Model file for the job. Use its own axes, mm. Give positions to 0.01 mm unless a question says otherwise; leave off trailing zeros. Write each loop counter-clockwise with the first axis right and the second up, starting at its lowest first coordinate (ties: lowest second). Pieces come first, ordered by that corner, then holes. Notation, with made-up numbers: (54.25, 40.5) - (92.25, 40.5) arc R32 ccw to (92.25, 74.5) - close; hole circle Ø10 at (12, 75.25). An arc over 180 degrees is marked (long way). Use CSV: the item, a comma, the result in double quotes.
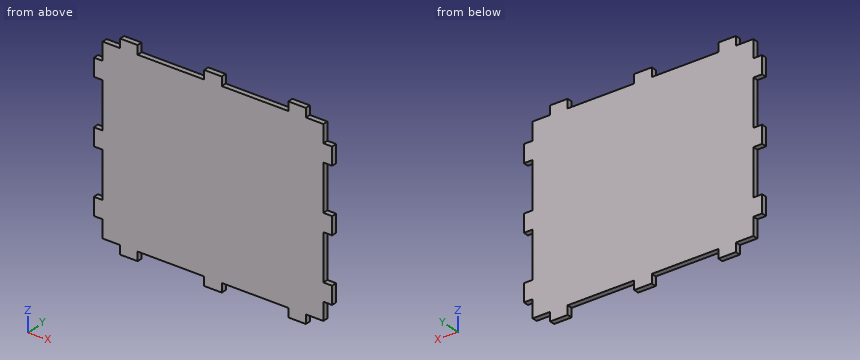
from build123d import *

# Parameters (mm, degrees)
F0_W     = 6.35
F0_H     = 12.7
F0_W_2   = 12.7
F0_H_2   = 6.35
F1_DEPTH = 3.81


# Not quite as in the source:
# - a feature names something its author has since deleted; it is built from what else it names


with BuildPart() as f1:
    # F0 (on Front) → F1 (new body)
    with BuildSketch(Plane.XZ):
        with Locations((-354.6769669852, 49.3793434303)):
            Rectangle(F0_W, F0_H)
        with Locations((-361.0269669852, 49.3793434303)):
            Rectangle(F0_W, F0_H)
        Polygon((-332.4519669852, -61.5706565697), (-284.2019669852, -61.5706565697), (-284.2019669852, -55.2206565697), (-277.8519669852, -55.2206565697), (-277.8519669852, 62.0793434303), (-284.2019669852, 62.0793434303), (-284.2019669852, 68.4293434303), (-332.4519669852, 68.4293434303), (-332.4519669852, 62.0793434303), (-345.1519669852, 62.0793434303), (-345.1519669852, 68.4293434303), (-357.8519669852, 68.4293434303), (-357.8519669852, 55.7293434303), (-351.5019669852, 55.7293434303), (-351.5019669852, 43.0293434303), (-357.8519669852, 43.0293434303), (-357.8519669852, 9.7793434303), (-351.5019669852, 9.7793434303), (-351.5019669852, -2.9206565697), (-357.8519669852, -2.9206565697), (-357.8519669852, -36.1706565697), (-351.5019669852, -36.1706565697), (-351.5019669852, -48.8706565697), (-357.8519669852, -48.8706565697), (-357.8519669852, -61.5706565697), (-345.1519669852, -61.5706565697), (-345.1519669852, -55.2206565697), (-332.4519669852, -55.2206565697), align=None)
        with Locations((-338.8019669852, 65.2543434303)):
            Rectangle(F0_W_2, F0_H_2)
        with Locations((-338.8019669852, 71.6043434303)):
            Rectangle(F0_W_2, F0_H_2)
        Polygon((-210.5519669852, -61.5706565697), (-197.8519669852, -61.5706565697), (-197.8519669852, -48.8706565697), (-204.2019669852, -48.8706565697), (-204.2019669852, -36.1706565697), (-197.8519669852, -36.1706565697), (-197.8519669852, -2.9206565697), (-204.2019669852, -2.9206565697), (-204.2019669852, 9.7793434303), (-197.8519669852, 9.7793434303), (-197.8519669852, 43.0293434303), (-204.2019669852, 43.0293434303), (-204.2019669852, 55.7293434303), (-197.8519669852, 55.7293434303), (-197.8519669852, 68.4293434303), (-210.5519669852, 68.4293434303), (-210.5519669852, 62.0793434303), (-223.2519669852, 62.0793434303), (-223.2519669852, 68.4293434303), (-271.5019669852, 68.4293434303), (-271.5019669852, 62.0793434303), (-277.8519669852, 62.0793434303), (-277.8519669852, -55.2206565697), (-271.5019669852, -55.2206565697), (-271.5019669852, -61.5706565697), (-223.2519669852, -61.5706565697), (-223.2519669852, -55.2206565697), (-210.5519669852, -55.2206565697), align=None)
        Polygon((-284.2019669852, 68.4293434303), (-277.8519669852, 68.4293434303), (-271.5019669852, 68.4293434303), (-271.5019669852, 74.7793434303), (-284.2019669852, 74.7793434303), align=None)
        with Locations((-274.6769669852, 65.2543434303)):
            Rectangle(F0_W, F0_H_2)
        with Locations((-281.0269669852, 65.2543434303)):
            Rectangle(F0_W, F0_H_2)
        with Locations((-216.9019669852, 71.6043434303)):
            Rectangle(F0_W_2, F0_H_2)
        with Locations((-216.9019669852, 65.2543434303)):
            Rectangle(F0_W_2, F0_H_2)
        with Locations((-354.6769669852, 3.4293434303)):
            Rectangle(F0_W, F0_H)
        with Locations((-361.0269669852, 3.4293434303)):
            Rectangle(F0_W, F0_H)
        with Locations((-361.0269669852, -42.5206565697)):
            Rectangle(F0_W, F0_H)
        with Locations((-338.8019669852, -64.7456565697)):
            Rectangle(F0_W_2, F0_H_2)
        with Locations((-354.6769669852, -42.5206565697)):
            Rectangle(F0_W, F0_H)
        with Locations((-338.8019669852, -58.3956565697)):
            Rectangle(F0_W_2, F0_H_2)
        with Locations((-281.0269669852, -58.3956565697)):
            Rectangle(F0_W, F0_H_2)
        with Locations((-274.6769669852, -58.3956565697)):
            Rectangle(F0_W, F0_H_2)
        Polygon((-271.5019669852, -67.9206565697), (-271.5019669852, -61.5706565697), (-277.8519669852, -61.5706565697), (-284.2019669852, -61.5706565697), (-284.2019669852, -67.9206565697), align=None)
        with Locations((-216.9019669852, -64.7456565697)):
            Rectangle(F0_W_2, F0_H_2)
        with Locations((-216.9019669852, -58.3956565697)):
            Rectangle(F0_W_2, F0_H_2)
        with Locations((-201.0269669852, -42.5206565697)):
            Rectangle(F0_W, F0_H)
        with Locations((-194.6769669852, -42.5206565697)):
            Rectangle(F0_W, F0_H)
        with Locations((-201.0269669852, 3.4293434303)):
            Rectangle(F0_W, F0_H)
        with Locations((-194.6769669852, 3.4293434303)):
            Rectangle(F0_W, F0_H)
        with Locations((-201.0269669852, 49.3793434303)):
            Rectangle(F0_W, F0_H)
        with Locations((-194.6769669852, 49.3793434303)):
            Rectangle(F0_W, F0_H)
    extrude(amount=F1_DEPTH)


solid = f1.part
(1) Saw through at A-A, the plane z = -17. List the corners of the cut face in (x, y), then the cut area to 3 significant figures.
Checked values:
outline,"(-357.85, -3.81) - (-197.85, -3.81) - (-197.85, 0) - (-357.85, 0) - close"
area,"610 mm^2"
(2) Flat gauge pins, fed straight in: P1, Ø1.9, axis at y = -2, z = 72.5, coming from the +X side; P2, Ø1.9, axis at y = -2, z = -54.5, coming from the +X side; P3, Ø1.1, axis at y = -2.5, z = -64, coming from the -X side. Where does each tip first touch, or does it go through?
Checked values:
P1,"stops at x = -210.55"
P2,"stops at x = -197.85"
P3,"stops at x = -345.15"
(3) Saw through at B-B, the plane x = -290. List the corners of the cut face in (y, z).
Checked values:
outline,"(-3.81, -61.57) - (0, -61.57) - (0, 68.43) - (-3.81, 68.43) - close"
(4) Wall check: probe 1 along Z at (x, y) = (-346, -3.15); probe 2 along X at (y, z) = (-0.2, -13). Give the ranges that are in metal, low to high. Write a range as [from, to].
Checked values:
probe 1,"z = [-61.57, 68.43]"
probe 2,"x = [-357.85, -197.85]"
